from build123d import *

# Parameters (mm, degrees)
SKETCH_1_W          = 60
SKETCH_1_H          = 131
EXTRUDE_1_DEPTH     = 5
SKETCH_2_W          = 30
SKETCH_2_H          = 131
EXTRUDE_2_DEPTH     = 6
SKETCH_3_R          = 20
CUT_EXTRUDE_1_DEPTH = 10
CHAMFER_1_SIZE      = 2
FILLET_1_R          = 3
SKETCH_13_R         = 1.6
CUT_EXTRUDE_2_DEPTH = 6
SKETCH_14_R         = 3
CUT_EXTRUDE_3_DEPTH = 3
CHAMFER_4_SIZE      = 1
SKETCH_16_W         = 50
SKETCH_16_H         = 6
EXTRUDE_4_DEPTH     = 25
FILLET_3_R          = 4
FILLET_4_R          = 10
FILLET_5_R          = 8
CUT_EXTRUDE_4_DEPTH = 4
FILLET_6_R          = 6
SKETCH_19_R         = 2.2
CUT_EXTRUDE_5_DEPTH = 18
SKETCH_20_R         = 2.2
CUT_EXTRUDE_6_DEPTH = 18


with BuildPart() as part:
    # 草图1 → 凸台-拉伸1 (new body)
    with BuildSketch(Plane.XY):
        with Locations((-207.175860782, 60.5)):
            Rectangle(SKETCH_1_W, SKETCH_1_H)
    extrude(amount=EXTRUDE_1_DEPTH)

    # 草图2 → 凸台-拉伸2 (add)
    with BuildSketch(Plane.ZY.offset(237.175860782)):
        with Locations((-10, 60.5)):
            Rectangle(SKETCH_2_W, SKETCH_2_H)
    extrude(amount=EXTRUDE_2_DEPTH)

    # 草图3 → 切除-拉伸1 (cut)
    with BuildSketch(Plane.XY.offset(5)):
        with Locations((-207.675860782, 60.5)):
            Circle(SKETCH_3_R)
    extrude(amount=-CUT_EXTRUDE_1_DEPTH, mode=Mode.SUBTRACT)

    # 倒角1
    chamfer_1_edges = [part.edges().sort_by_distance(p)[0] for p in [
        (-243.175860782, 60.5, 5),
    ]]
    chamfer(chamfer_1_edges, length=CHAMFER_1_SIZE)

    # 圆角1
    fillet_1_edges = [part.edges().sort_by_distance(p)[0] for p in [
        (-240.175860782, 126, -25),
        (-240.175860782, -5, -25),
        (-177.175860782, 126, 2.5),
        (-177.175860782, -5, 2.5),
    ]]
    fillet(fillet_1_edges, radius=FILLET_1_R)

    # 草图13 → 切除-拉伸2 (cut)
    with BuildSketch(Plane.XY.offset(5)):
        with Locations((-207.675860782, 85.5)):
            Circle(SKETCH_13_R)
        with Locations((-229.326495877, 73)):
            Circle(SKETCH_13_R)
        with Locations((-186.025225688, 73)):
            Circle(SKETCH_13_R)
        with Locations((-186.025225688, 48)):
            Circle(SKETCH_13_R)
        with Locations((-207.675860782, 35.5)):
            Circle(SKETCH_13_R)
        with Locations((-229.326495877, 48)):
            Circle(SKETCH_13_R)
    extrude(amount=-CUT_EXTRUDE_2_DEPTH, mode=Mode.SUBTRACT)

    # 草图14 → 切除-拉伸3 (cut)
    with BuildSketch(Plane.XY.offset(5)):
        with Locations((-207.675860782, 85.5)):
            Circle(SKETCH_14_R)
        with Locations((-186.025225688, 73)):
            Circle(SKETCH_14_R)
        with Locations((-186.025225688, 48)):
            Circle(SKETCH_14_R)
        with Locations((-207.675860782, 35.5)):
            Circle(SKETCH_14_R)
        with Locations((-229.326495877, 48)):
            Circle(SKETCH_14_R)
        with Locations((-229.326495877, 73)):
            Circle(SKETCH_14_R)
    extrude(amount=-CUT_EXTRUDE_3_DEPTH, mode=Mode.SUBTRACT)

    # 倒角4
    chamfer_4_edges = [part.edges().sort_by_distance(p)[0] for p in [
        (-243.175860782, 126, -9.5),
        (-242.175860782, 126, 4),
        (-210.675860782, -5, 5),
        (-242.175860782, -5, 4),
        (-243.175860782, 60.5, -25),
        (-210.675860782, 126, 5),
        (-243.175860782, -5, -9.5),
        (-243.175860782, -4.121320344, -24.121320344),
        (-243.175860782, 125.121320344, -24.121320344),
        (-177.175860782, 60.5, 5),
        (-178.054540439, -4.121320344, 5),
        (-178.054540439, 125.121320344, 5),
    ]]
    chamfer(chamfer_4_edges, length=CHAMFER_4_SIZE)

    # 草图16 → 凸台-拉伸4 (add)
    with BuildSketch(Plane(origin=(0, 0, 0), x_dir=(-1, 0, 0), z_dir=(0, 0, -1))):
        with Locations((212.175860782, 117)):
            Rectangle(SKETCH_16_W, SKETCH_16_H)
    extrude_4 = extrude(amount=EXTRUDE_4_DEPTH)

    # 镜向1: 凸台-拉伸4 across plane
    add(extrude_4.mirror(Plane(origin=(0, 60.5, 0), x_dir=(0, 0, 1), z_dir=(0, -1, 0))))

    # 圆角3
    fillet_3_edges = [part.edges().sort_by_distance(p)[0] for p in [
        (-237.175860782, -2, 0),
        (-237.175860782, 123, 0),
    ]]
    fillet(fillet_3_edges, radius=FILLET_3_R)

    # 圆角4
    fillet_4_edges = [part.edges().sort_by_distance(p)[0] for p in [
        (-237.175860782, 114, -12.5),
        (-237.175860782, 7, -12.5),
    ]]
    fillet(fillet_4_edges, radius=FILLET_4_R)

    # 圆角5
    fillet_5_edges = [part.edges().sort_by_distance(p)[0] for p in [
        (-187.175860782, 117, -25),
        (-187.175860782, 117, 0),
        (-187.175860782, 4, 0),
        (-187.175860782, 4, -25),
    ]]
    fillet(fillet_5_edges, radius=FILLET_5_R)

    # 草图17 → 切除-拉伸4 (cut)
    with BuildSketch(Plane(origin=(0, 120, 0), x_dir=(1, 0, 0), z_dir=(0, 1, 0))):
        with BuildLine():
            Line((-235.175860782, 4), (-235.175860782, 2))
            Line((-235.175860782, 2), (-233.175860782, 2))
            Line((-233.175860782, 2), (-187.175860782, 2))
            ThreePointArc((-187.175860782, 2), (-188.662693763, 4.83772234), (-189.175860782, 8))
            Line((-189.175860782, 8), (-189.175860782, 17))
            ThreePointArc((-189.175860782, 17), (-190.933220095, 21.242640687), (-195.175860782, 23))
            Line((-195.175860782, 23), (-235.175860782, 23))
            Line((-235.175860782, 23), (-235.175860782, 4))
        make_face()
    cut_extrude_4 = extrude(amount=-CUT_EXTRUDE_4_DEPTH, mode=Mode.SUBTRACT)

    # 镜向2: 切除-拉伸4 across plane
    add(cut_extrude_4.mirror(Plane(origin=(0, 60.5, 0), x_dir=(0, 0, 1), z_dir=(0, -1, 0))), mode=Mode.SUBTRACT)

    # 圆角6
    fillet_6_edges = [part.edges().sort_by_distance(p)[0] for p in [
        (-187.175860782, 118, -2),
        (-235.175860782, 118, -23),
        (-235.175860782, 118, -2),
        (-235.175860782, 3, -23),
        (-187.175860782, 3, -2),
        (-235.175860782, 3, -2),
    ]]
    fillet(fillet_6_edges, radius=FILLET_6_R - 0.0001)  # a hair under: the kernel refuses the full size

    # 草图19 → 切除-拉伸5 (cut)
    with BuildSketch(Plane.XY.offset(5)):
        with Locations((-217.175860782, -2)):
            Circle(SKETCH_19_R)
        with Locations((-187.175860782, -2)):
            Circle(SKETCH_19_R)
        with Locations((-197.175860782, -2)):
            Circle(SKETCH_19_R)
        with Locations((-207.175860782, -2)):
            Circle(SKETCH_19_R)
        with Locations((-227.175860782, -2)):
            Circle(SKETCH_19_R)
    cut_extrude_5 = extrude(amount=-CUT_EXTRUDE_5_DEPTH, mode=Mode.SUBTRACT)

    # 镜向3: 切除-拉伸5 across plane
    add(cut_extrude_5.mirror(Plane(origin=(0, 60.5, 0), x_dir=(0, 0, 1), z_dir=(0, -1, 0))), mode=Mode.SUBTRACT)

    # 草图20 → 切除-拉伸6 (cut)
    with BuildSketch(Plane.ZY.offset(243.175860782)):
        with Locations((-20.5, -2)):
            Circle(SKETCH_20_R)
        with Locations((-13, -2)):
            Circle(SKETCH_20_R)
    cut_extrude_6 = extrude(amount=-CUT_EXTRUDE_6_DEPTH, mode=Mode.SUBTRACT)

    # 镜向4: 切除-拉伸6 across plane
    add(cut_extrude_6.mirror(Plane(origin=(0, 60.5, 0), x_dir=(0, 0, 1), z_dir=(0, -1, 0))), mode=Mode.SUBTRACT)


solid = part.part
Source: CAD feature listing. Evaluate the final solid. Frame: model axes, mm. A direction names the side the tool comes from. Give positions to 0.01 mm unless a question says otherwise; leave off trailing zeros. Order: outer loops, then holes, each group sorted by start corner. A loop starts at its lowest first (then second) coordinate and runs counter-clockwise, first axis right, second up. Notation, with made-up numbers: (71.25, 46) -> (124.25, 46) arc R23 ccw to (124.25, 82) -> close; hole circle Ø3 at (-16, 25). An arc over 180 degrees is marked (long way). Use a Markdown table: item, result.
1) Ray query, line 1 along X through (y, z) = (123, 3); line 2 along Y through (x, z) = (-238.4, -20.5); line 3 along Y through (x, z) = (-216, -22.5). Return the intervals inside material, ascending. Write a range as [from, to].
Answer list:
| item | result |
|---|---|
| line 1 | [-243.18, -229.38], [-224.98, -219.38], [-214.98, -209.38], [-204.98, -199.38], [-194.98, -189.38], [-184.98, -177.18] |
| line 2 | [-5, -4.2], [0.2, 120.8], [125.2, 126] |
| line 3 | [5, 7], [114, 116] |
2) Reachability of faces 1 (the flat face through (-194, 76, 0)), 2 (the flat face through (-212, 3, -23)), 3 (the flat face through (-237.176, 0, -15)), 4 (the cylindrical face through (-204.814, 36.401, 3.521)), 5 (the cylindrical face through (-190.89, 118.03, -21.2)) from +Z, -Z, +X, -X, +Y, -Y: full face, straight path, thin tool, end or side. Return the list, or none.
Answer list:
| item | result |
|---|---|
| face 1 | -Z, +X |
| face 2 | -Y |
| face 3 | -Z, +X, -Y |
| face 4 | +Z |
| face 5 | +Y |
3) Contact query for flat-ended pins moving along their axis: P1, Ø3.5, axis at x = -186.03, y = 48, coming from the +Z side; P2, Ø4, axis at y = 15, z = -16, coming from the +X side; P3, Ø4.5, axis at y = 2, z = -10.5, coming from the +X side. Output: stop coordinate, or through.
Answer list:
| item | result |
|---|---|
| P1 | z = 2 |
| P2 | x = -236.34 |
| P3 | x = -187.18 |
4) Section query A-A, the plane y = 85.5. Return the cut outline in (x, z), then the cut area to 3 significant figures.
Answer list:
| item | result |
|---|---|
| outline | (-243.18, -24) -> (-242.18, -25) -> (-237.18, -25) -> (-237.18, 0) -> (-209.28, 0) -> (-209.28, 2) -> (-210.68, 2) -> (-210.68, 5) -> (-241.18, 5) -> (-243.18, 3) -> close; (-206.08, 0) -> (-177.18, 0) -> (-177.18, 4) -> (-178.18, 5) -> (-204.68, 5) -> (-204.68, 2) -> (-206.08, 2) -> close |
| area | 453 mm² |
5) Section query B-B, the plane x = -221. Return the cut outline in (y, z), then the cut area to 3 significant figures.
Answer list:
| item | result |
|---|---|
| outline | (-5, 0) -> (1, 0) -> (1, -2) -> (5, -2) -> (5, -23) -> (1, -23) -> (1, -25) -> (7, -25) -> (7, 0) -> (45.58, 0) -> (45.58, 5) -> (-4, 5) -> (-5, 4) -> close; (75.42, 0) -> (114, 0) -> (114, -25) -> (120, -25) -> (120, -23) -> (116, -23) -> (116, -2) -> (120, -2) -> (120, 0) -> (126, 0) -> (126, 4) -> (125, 5) -> (75.42, 5) -> close |
| area | 637 mm² |
6) Section query C-C, the plane y = 23.5. Return the cut outline in (x, z), then the cut area to 3 significant figures.
Answer list:
| item | result |
|---|---|
| outline | (-243.18, -24) -> (-242.18, -25) -> (-237.18, -25) -> (-237.18, 0) -> (-177.18, 0) -> (-177.18, 4) -> (-178.18, 5) -> (-241.18, 5) -> (-243.18, 3) -> close |
| area | 477 mm² |
7) Mould query, pull axis Z, two halves, no side actions, for faces 6 (the flat face through (-212, 5, -13)), 7 (the flat face through (-228, 71.7, 2)), 8 (the flat face through (-208, 7, -12)), 9 (the cylindrical face through (-239.71, -4.14, -24.1)). Classes: +Z half, -Z half, draft (parallel to the pull), parting line (faces both ways), or undercut.
Answer list:
| item | result |
|---|---|
| face 6 | undercut |
| face 7 | +Z half |
| face 8 | draft |
| face 9 | -Z half |
8) Section query D-D, the plane x = -212. Return the cut outline in (y, z).
Answer list:
| item | result |
|---|---|
| outline | (-5, 0) -> (1, 0) -> (1, -2) -> (5, -2) -> (5, -23) -> (1, -23) -> (1, -25) -> (7, -25) -> (7, 0) -> (40.97, 0) -> (40.97, 5) -> (-4, 5) -> (-5, 4) -> close; (80.03, 0) -> (114, 0) -> (114, -25) -> (120, -25) -> (120, -23) -> (116, -23) -> (116, -2) -> (120, -2) -> (120, 0) -> (126, 0) -> (126, 4) -> (125, 5) -> (80.03, 5) -> close |
